```python
from build123d import *

# Parameters (mm, degrees)
SKETCH_1_R          = 3
EXTRUDE_1_DEPTH     = 44
SKETCH_2_R          = 1.2
CUT_EXTRUDE_1_DEPTH = 44
FILLET_1_R          = 1
FILLET_2_R          = 0.3


with BuildPart() as part:
    # 草图1 → 凸台-拉伸1 (new body)
    with BuildSketch(Plane(origin=(0, 0, 0), x_dir=(0, 0, -1), z_dir=(1, 0, 0))):
        Circle(SKETCH_1_R)
    extrude(amount=EXTRUDE_1_DEPTH)

    # 草图2 → 切除-拉伸1 (cut)
    with BuildSketch(Plane.ZY):
        Circle(SKETCH_2_R)
    extrude(amount=-CUT_EXTRUDE_1_DEPTH, mode=Mode.SUBTRACT)

    # 圆角1
    fillet_1_edges = [part.edges().sort_by_distance(p)[0] for p in [
        (0, 0, 3),
        (44, 0, 3),
    ]]
    fillet(fillet_1_edges, radius=FILLET_1_R)

    # 圆角2
    fillet_2_edges = [part.edges().sort_by_distance(p)[0] for p in [
        (44, 0, -1.2),
        (0, 0, -1.2),
    ]]
    fillet(fillet_2_edges, radius=FILLET_2_R)


solid = part.part
```
Could you check a few things on this model? Use its own coordinates, in mm. Coordinates: 2 decimals unless noted, no trailing zeros. Write each loop counter-clockwise with the first axis right and the second up, starting at its lowest first coordinate (ties: lowest second). Pieces come first, ordered by that corner, then holes. Notation, with made-up numbers: M 69,44.25 L 111,44.25 A24 cw 111,72.25 Z; hole C 71.25,8.25 d10. An arc over 180 degrees is marked long. Answer as CSV lines item,"result". Start each with the question number.
1) For P1, Ø1, axis at x = 36, y = -1, coming from the -Z side; P2, Ø1, axis at x = 6, z = 1, coming from the -Y side; P3, Ø1.5, axis at x = 24.5, z = 1.5, coming from the +Y side, each with a flat end and sliding along its axis, tell me the tip position at first contact or that it passes through.
2) We'd pull the mould along Z, two halves only. Please class faces 1 (the cylindrical face through (21.7, 1.01, 0.65)), 2 (the cylindrical face through (22, 0, 3)): +Z half, -Z half, draft (parallel to the pull), parting line (faces both ways), or undercut.
3) Please list where these lines run through material, in increasing order: line 1 (Y direction, x = 16, z = 0); line 2 (Y direction, x = 14.5, z = -0.5); line 3 (Z direction, x = 30, y = 2.75). Write a range as from..to.
4) I want a section at C-C, the plane x = 12. Please give me the cut outline in (y, z), and give its area (3 significant figures).
5) I want a section at A-A, the plane z = 0. Please give me the cut outline in (x, y), and give its area (3 significant figures).
Data:
1,P1,"stops at z = -2.96"
1,P2,"stops at y = -2.96"
1,P3,"stops at y = 2.9"
2,face 1,"undercut"
2,face 2,"parting line"
3,line 1,"y = -3..-1.2, 1.2..3"
3,line 2,"y = -2.96..-1.09, 1.09..2.96"
3,line 3,"z = -1.2..1.2"
4,outline,"C 0,0 d6; hole C 0,0 d2.4"
4,area,"23.8 mm^2"
5,outline,"M 0,-2 A1 ccw 1,-3 L 43,-3 A1 ccw 44,-2 L 44,-1.5 A0.3 ccw 43.7,-1.2 L 0.3,-1.2 A0.3 ccw 0,-1.5 Z; M 0,1.5 A0.3 ccw 0.3,1.2 L 43.7,1.2 A0.3 ccw 44,1.5 L 44,2 A1 ccw 43,3 L 1,3 A1 ccw 0,2 Z"
5,area,"157 mm^2"
